Could you check a few things on this drawing? It's one solid part, dimensions in mm from its lowest x, y, z. Round coordinates to 2 decimals unless told otherwise and drop trailing zeros. Loops run counter-clockwise (first coordinate to the right, second up) from the corner with the lowest first, then second, coordinate; pieces in that order, holes last. Notation, with made-up numbers: M 84.25,18.5 L 143.25,18.5 A10 cw 143.25,25.5 Z; hole C -22.5,23 d11. An arc over 180 degrees is marked long. Answer as CSV lines item,"result".
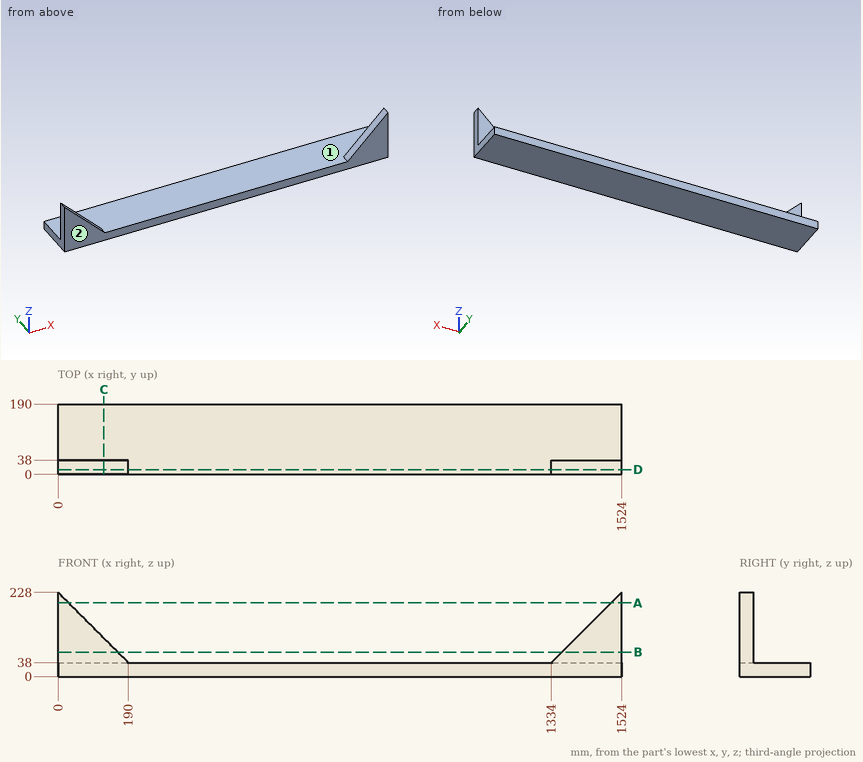
Item 1: We'd pull the mould along X, two halves only. Please class the marked faces 1 and 2: released by +X, released by -X, zero draft, split by the parting line, or undercut.
Output:
face 1,"undercut"
face 2,"zero draft"
Item 2: If we section it at A-A on z = 199.5: Write out the boundary of the cut face in (x, y).
Output:
outline,"M 0,0 L 28.5,0 L 28.5,38 L 0,38 Z; M 1495.5,0 L 1524,0 L 1524,38 L 1495.5,38 Z"
Item 3: If I drill on line 1 along Z through (x, y) = (436.5, 78.5); line 2 along X through (y, z) = (33.5, 131), over which ranges is the centre line in solid material (lowest first)? Write a range as from..to.
Output:
line 1,"z = 0..38"
line 2,"x = 0..97, 1427..1524"
Item 4: If we section it at B-B on z = 66: Write out the boundary of the cut face in (x, y), then the cut area to 3 significant figures.
Output:
outline,"M 0,0 L 162,0 L 162,38 L 0,38 Z; M 1362,0 L 1524,0 L 1524,38 L 1362,38 Z"
area,"12,300 mm2"
Item 5: If we section it at D-D on y = 12.5: Write out the boundary of the cut face in (x, z), then the cut area to 3 significant figures.
Output:
outline,"M 0,0 L 1524,0 L 1524,228 L 1334,38 L 190,38 L 0,228 Z"
area,"94,000 mm2"
Item 6: If we section it at C-C on x = 124: Write out the boundary of the cut face in (y, z).
Output:
outline,"M 0,0 L 190,0 L 190,38 L 38,38 L 38,104 L 0,104 Z"
